Check sheet for the modelled part. Datum: model origin and axes. Units: mm. A direction names the side the tool comes from. Give positions to 0.01 mm unless a question says otherwise; leave off trailing zeros. Loops run counter-clockwise (first coordinate to the right, second up) from the corner with the lowest first, then second, coordinate; pieces in that order, holes last. Notation, with made-up numbers: M -33,37 L 8,37 A20 ccw 8,60 Z; hole C 9.25,71.25 d2. An arc over 180 degrees is marked long. Put each result on its own line as item: value. Start each with the question number.
Autodesk Inventor part; units mm, degrees
ref_plane "YZ Plane" through (0, 0, 0) normal (1, 0, 0) x (0, 1, 0)
ref_plane "XZ Plane" through (0, 0, 0) normal (0, 1, 0) x (-1, 0, 0)
ref_plane "XY Plane" through (0, 0, 0) normal (0, 0, 1) x (1, 0, 0)
sketch "スケッチ1" plane through (0, 0, 0) normal (0, 0, 1) x (1, 0, 0)
  line L0 (-22.5, 3.5) -> (22.5, 3.5)
  line L1 (22.5, 3.5) -> (22.5, -3.5)
  line L2 (22.5, -3.5) -> (-22.5, -3.5)
  line L3 (-22.5, -3.5) -> (-22.5, 3.5)
  line L4 (-22.5, 3.5) -> (22.5, -3.5) construction
  line L5 (22.5, 3.5) -> (-22.5, -3.5) construction
  line L6 (0, -6.37) -> (0, 6.37) construction
  line L7 (-34.37, 0) -> (34.37, 0) construction
  circle A0 centre (-20, 0) radius 4.55
  line L8 (22.5, -3.5) -> (22.5, 3.5)
  circle A1 centre (20, 0) radius 4.55
  circle A2 centre (-20, 0) radius 1.635
  circle A3 centre (20, 0) radius 1.635
  line L9 (14, 3.5) -> (14, -3.5)
  line L10 (16, 3.5) -> (16, -3.5)
  point P0 (0, 0)
  point P1 (-17.0927, 3.5)
  point P2 (-22.9073, 3.5)
  point P3 (-22.9073, -3.5)
  point P4 (-17.0927, -3.5)
  point P5 (17.0927, 3.5)
  point P6 (17.0927, -3.5)
  point P7 (22.9073, -3.5)
  point P8 (22.9073, 3.5)
  dimension "d1" = 7
  dimension "d2" = 20
  dimension "d3" = 45
  dimension "d4" = 9.1
  dimension "d12" = 3.27
  dimension "d13" = 3.27
  dimension "d14" = 6
  dimension "d15" = 2
extrude "押し出し1" add sketch "スケッチ1" along normal mid plane 5 contours L9 L2 A0 L0 | L0 L10 A1 L2 L9 | L0 A1 L10 | A0 L2 L3 L0 | L0 L1 L2 A1 L10 | L10 A1 | L10 A1 L2 picked at (-19.7985, 2.8744)
fillet "フィレット1" radius 3 4 edges at (-22.5, 3.5, 0) (-22.5, -3.5, 0) (22.5, -3.5, 0) (22.5, 3.5, 0)
extrude "押し出し3" add sketch "スケッチ1" along normal mid plane 11 contours L0 L10 A1 L2 L9 | L0 A1 L10 | L0 L1 L2 A1 L10 | L10 A1 | L10 A1 L2
extrude "押し出し4" cut sketch "スケッチ1" along normal mid plane 7 contours L0 A1 L10 | L0 L1 L2 A1 L10 | L10 A1 L2
fillet "フィレット2" radius 3 8 edges at (22.5, 3.5, 4.5) (22.5, -3.5, 4.5) (22.5, 3.5, -4.5) (22.5, -3.5, -4.5) (14, 3.5, 4) (14, -3.5, 4) (14, 3.5, -4) (14, -3.5, -4)
properties part number "link_arm_1"
Q1. Section check A-A, the plane y = 0. Record the cut outline in (x, z) (3 decimals).
Q2. Section check D-D, the plane x = -20. Record the cut outline in (y, z) (3 decimals).
Q3. Access from +Z, -Z, +X, -X, +Y, -Y to the whole of each face (thin tool, end or side, straight path). Record for faces 4 (the face through (14.86, 2.6, -4.02)), 5 (the face through (14, 0, 4)), 6 (the face through (14, 0, -4)), 7 (the face through (16, 0, 0)), 8 (the face through (14.86, 2.6, 3.98)).
Q4. Section check B-B, the plane z = -1.5. Record the cut outline in (x, y) (3 decimals), then the cut area to 3 significant figures.
Q5. Mould release check, pull along Z, two halves, no side actions. Record for faces 1 (the face through (18, 0, -5.5)), 2 (the face through (-2, 3.5, 0)), 3 (the face through (18, 1, -3.5)): pulls with the +Z half, pulls with the -Z half, needs draft (parallel to the pull), parting line crosses it, or undercut.
Q6. Section check C-C, the plane x = 20. Record the cut outline in (y, z) (3 decimals).
Q7. Thickness scan on line 1 along Z through (x, y) = (-6, -2.5); line 2 along Y through (x, z) = (-20, 1) (3 decimals); line 3 along X through (y, z) = (1, -3.75). Record the ranges inside material, lowest first. Write a range as [from, to].
Q8. Depth check by flat-ended pin: P1, Ø4, axis at x = -20, y = 0, coming from the -Z side; P2, Ø0.5, axis at y = 0, z = -4, coming from the -X side; P3, Ø2, axis at x = 20, y = 0, coming from the +Z side; P4, Ø1, axis at y = 2.5, z = -1.5, coming from the +X side. Enter the tip coordinate at first touch or a pass-through.
Found:
1. outline: M -22.5,-2.5 L -21.635,-2.5 L -21.635,2.5 L -22.5,2.5 Z; M -18.365,-2.5 L 14,-2.5 L 14,-5.5 L 18.365,-5.5 L 18.365,-3.5 L 16,-3.5 L 16,3.5 L 18.365,3.5 L 18.365,5.5 L 14,5.5 L 14,2.5 L -18.365,2.5 Z; M 21.635,-5.5 L 22.5,-5.5 L 22.5,-3.5 L 21.635,-3.5 Z; M 21.635,3.5 L 22.5,3.5 L 22.5,5.5 L 21.635,5.5 Z
2. outline: M -3.458,-2.5 L -1.635,-2.5 L -1.635,2.5 L -3.458,2.5 Z; M 1.635,-2.5 L 3.458,-2.5 L 3.458,2.5 L 1.635,2.5 Z
3. face 4: -Z, -X, +Y
3. face 5: +Z, -X, +Y, -Y
3. face 6: -Z, -X, +Y, -Y
3. face 7: +X, +Y, -Y
3. face 8: +Z, -X, +Y
4. outline: M -22.5,-0.5 A3 ccw -19.5,-3.5 L 16,-3.5 L 16,3.5 L -19.5,3.5 A3 ccw -22.5,0.5 Z; hole C -20,0 d3.27
4. area: 257 mm^2
5. face 1: pulls with the -Z half
5. face 2: needs draft
5. face 3: undercut
6. outline: M -3.458,-5.5 L -1.635,-5.5 L -1.635,-3.5 L -3.458,-3.5 Z; M -3.458,3.5 L -1.635,3.5 L -1.635,5.5 L -3.458,5.5 Z; M 1.635,-5.5 L 3.458,-5.5 L 3.458,-3.5 L 1.635,-3.5 Z; M 1.635,3.5 L 3.458,3.5 L 3.458,5.5 L 1.635,5.5 Z
7. line 1: z = [-2.5, 2.5]
7. line 2: y = [-3.458, -1.635], [1.635, 3.458]
7. line 3: x = [14.04, 18.71], [21.29, 22.46]
8. P1: stops at z = -2.5
8. P2: stops at x = 14
8. P3: passes through
8. P4: stops at x = 16
